```python
from build123d import *

# Parameters (mm, degrees)
SKETCH_1_W      = 125
SKETCH_1_H      = 72.5
SKETCH_1_R      = 5.1
SKETCH_1_R_2    = 2.1
EXTRUDE_1_DEPTH = 3
CHAMFER_1_SIZE  = 30
CHAMFER_2_SIZE  = 4
CHAMFER_3_SIZE  = 2


with BuildPart() as part:
    # 草图1 → 凸台-拉伸1 (new, symmetric)
    with BuildSketch(Plane.XY):
        with Locations((0, -16.25)):
            Rectangle(SKETCH_1_W, SKETCH_1_H)
        Circle(SKETCH_1_R, mode=Mode.SUBTRACT)
        with Locations((-32.5, -42.5)):
            Circle(SKETCH_1_R_2, mode=Mode.SUBTRACT)
        with Locations((32.5, -42.5)):
            Circle(SKETCH_1_R_2, mode=Mode.SUBTRACT)
        with Locations((-52.5, -42.5)):
            Circle(SKETCH_1_R_2, mode=Mode.SUBTRACT)
        with Locations((52.5, -42.5)):
            Circle(SKETCH_1_R_2, mode=Mode.SUBTRACT)
        with Locations((-52.5, -22.5)):
            Circle(SKETCH_1_R_2, mode=Mode.SUBTRACT)
        with Locations((52.5, -22.5)):
            Circle(SKETCH_1_R_2, mode=Mode.SUBTRACT)
    extrude(amount=EXTRUDE_1_DEPTH, both=True)

    # 倒角1
    chamfer_1_edges = [part.edges().sort_by_distance(p)[0] for p in [
        (62.5, 20, 0),
        (-62.5, 20, 0),
    ]]
    chamfer(chamfer_1_edges, length=CHAMFER_1_SIZE)

    # 倒角2
    chamfer_2_edges = [part.edges().sort_by_distance(p)[0] for p in [
        (62.5, -52.5, 0),
        (-62.5, -52.5, 0),
    ]]
    chamfer(chamfer_2_edges, length=CHAMFER_2_SIZE)

    # 倒角3
    chamfer_3_edges = [part.edges().sort_by_distance(p)[0] for p in [
        (-54.6, -42.5, -3),
        (50.4, -42.5, -3),
        (-54.6, -22.5, -3),
        (50.4, -22.5, -3),
    ]]
    chamfer(chamfer_3_edges, length=CHAMFER_3_SIZE)


solid = part.part
```
The model under review builds one solid part; all positions refer to its coordinate system, in mm. Round coordinates to 2 decimals unless told otherwise and drop trailing zeros. Write each loop counter-clockwise with the first axis right and the second up, starting at its lowest first coordinate (ties: lowest second). Pieces come first, ordered by that corner, then holes.
(1) We need section C-C on y = -42.5. Give the boundary of the cut face in (x, z).
(2) Insertion check: pin 1 (3.5 mm diameter, centred on x = -52.5, y = -42.5, fed in from +Z); pin 2 (1 mm diameter, centred on y = -6.5, z = 2, fed in from -X); pin 3 (6.5 mm diameter, centred on x = -52.5, y = -22.5, fed in from -Z); pin 4 (5 mm diameter, centred on x = 52.5, y = -22.5, fed in from -Z). Each pin has a flat end and moves straight along its axis. Give the tip position at first contact, or say it passes through.
(3) We need section A-A on x = 52.5. Give the boundary of the cut face in (y, z), and give its area (3 significant figures).
(4) We need section D-D on z = 1. Give the boundary of the cut face in (x, y).
(5) Wall thickness on L1, parallel to Y at x = 0, z = -0.55; L2, parallel to Y at x = 52.5, z = 1.6; L3, parallel to Y at x = -54, z = 0: over which ranges is each line inside the solid? List them lowest first.
(6) Mouldability with a two-part tool opening along X and no side actions: class faces 1 (the flat face through (61, -50, 0)), 2 (the flat face through (-60, -51, 0)), 3 (the cylindrical face through (30.834, -43.778, -0.042)) as +X half, -X half, draft (parallel to the pull), parting line (faces both ways), or undercut.
(7) We need section B-B on y = -22.5. Give the boundary of the cut face in (x, z).
Findings below:
1. outline: (-62.5, -3) - (-56.6, -3) - (-54.6, -1) - (-54.6, 3) - (-62.5, 3) - close; (-50.4, -1) - (-48.4, -3) - (-34.6, -3) - (-34.6, 3) - (-50.4, 3) - close; (-30.4, -3) - (30.4, -3) - (30.4, 3) - (-30.4, 3) - close; (34.6, -3) - (48.4, -3) - (50.4, -1) - (50.4, 3) - (34.6, 3) - close; (54.6, -1) - (56.6, -3) - (62.5, -3) - (62.5, 3) - (54.6, 3) - close
2. pin 1: passes through
2. pin 2: stops at x = -59.5
2. pin 3: stops at z = -2.15
2. pin 4: stops at z = -1.4
3. outline: (-52.5, -3) - (-46.6, -3) - (-44.6, -1) - (-44.6, 3) - (-52.5, 3) - close; (-40.4, -1) - (-38.4, -3) - (-26.6, -3) - (-24.6, -1) - (-24.6, 3) - (-40.4, 3) - close; (-20.4, -1) - (-18.4, -3) - (0, -3) - (0, 3) - (-20.4, 3) - close
3. area: 257 mm2
4. outline: (-62.5, -48.5) - (-58.5, -52.5) - (58.5, -52.5) - (62.5, -48.5) - (62.5, -10) - (32.5, 20) - (-32.5, 20) - (-62.5, -10) - close; hole circle Ø4.2 at (-52.5, -42.5); hole circle Ø4.2 at (-52.5, -22.5); hole circle Ø4.2 at (-32.5, -42.5); hole circle Ø10.2 at (0, 0); hole circle Ø4.2 at (32.5, -42.5); hole circle Ø4.2 at (52.5, -42.5); hole circle Ø4.2 at (52.5, -22.5)
5. L1: y = -52.5 to -5.1, 5.1 to 20
5. L2: y = -52.5 to -44.6, -40.4 to -24.6, -20.4 to 0
5. L3: y = -52.5 to -43.97, -41.03 to -23.97, -21.03 to -1.5
6. face 1: +X half
6. face 2: -X half
6. face 3: undercut
7. outline: (-62.5, -3) - (-56.6, -3) - (-54.6, -1) - (-54.6, 3) - (-62.5, 3) - close; (-50.4, -1) - (-48.4, -3) - (48.4, -3) - (50.4, -1) - (50.4, 3) - (-50.4, 3) - close; (54.6, -1) - (56.6, -3) - (62.5, -3) - (62.5, 3) - (54.6, 3) - close
